Build history of the part. All positions in model axes, mm. A direction names the side the tool comes from. Round coordinates to 2 decimals unless told otherwise and drop trailing zeros. Write each loop counter-clockwise with the first axis right and the second up, starting at its lowest first coordinate (ties: lowest second). Pieces come first, ordered by that corner, then holes. Notation, with made-up numbers: (57, 75) -> (83, 75) arc R18 cw to (83, 108) -> close; hole circle Ø7 at (9.25, -37.5). An arc over 180 degrees is marked (long way). One line per question, with ' | ' between items.
from build123d import *

# Parameters (mm, degrees)
SKETCH3_W               = 36
SKETCH3_H               = 36
SKETCH3_W_2             = 20
SKETCH3_H_2             = 20
BOSS_EXTRUDE1_DEPTH     = 22
CUT_EXTRUDE1_REACH      = 57.462
SKETCH4_R               = 2.2
CUT_EXTRUDE2_DEPTH      = 56.461698495
CUT_EXTRUDE2_DEPTH_BACK = 56.461698495
SKETCH5_R               = 6.2
SKETCH6_W               = 22
SKETCH6_H               = 22
SKETCH6_R               = 6.7
BOSS_EXTRUDE2_DEPTH     = 5.4
SKETCH7_R               = 6.7
CUT_EXTRUDE3_DEPTH      = 5.4
SKETCH8_R               = 6.7
CUT_EXTRUDE4_DEPTH      = 5.4
SKETCH9_R               = 6.7
CUT_EXTRUDE5_DEPTH      = 5.4
FILLET2_R               = 2.5
FILLET3_R               = 2.5
FILLET4_R               = 2.5
SKETCH10_R              = 1.7
CUT_EXTRUDE6_DEPTH      = 56.461698535


with BuildPart() as part:
    # Sketch3 → Boss-Extrude1 (new body)
    with BuildSketch(Plane(origin=(0, 0, 0), x_dir=(1, 0, 0), z_dir=(0, 1, 0))):
        with Locations((18, -18)):
            Rectangle(SKETCH3_W, SKETCH3_H)
        with Locations((18, -18)):
            Rectangle(SKETCH3_W_2, SKETCH3_H_2, mode=Mode.SUBTRACT)
    extrude(amount=BOSS_EXTRUDE1_DEPTH)

    # Sketch4 → Cut-Extrude1 (cut, up to next)
    with BuildSketch(Plane(origin=(0, 0, 0), x_dir=(-1, 0, 0), z_dir=(0, 0, -1)), mode=Mode.PRIVATE) as cut_extrude1_sk1:
        with Locations((-16, 11)):
            Circle(SKETCH4_R)
    cut_extrude1_tool1 = extrude(cut_extrude1_sk1.sketch, amount=-CUT_EXTRUDE1_REACH, mode=Mode.PRIVATE) & part.part
    add(cut_extrude1_tool1.solids().sort_by_distance((16, 11, 0))[0], mode=Mode.SUBTRACT)

    # Sketch5 → Cut-Extrude2 (cut, two sides: drawn at the far end of the back side and taken through both)
    with BuildSketch(Plane(origin=(36, 0, 0), x_dir=(0, 0, -1), z_dir=(1, 0, 0)).offset(-CUT_EXTRUDE2_DEPTH_BACK)):
        with Locations(Location((-20, 11, 0), (0, 0, 180))):
            Circle(SKETCH5_R)
    extrude(amount=CUT_EXTRUDE2_DEPTH + CUT_EXTRUDE2_DEPTH_BACK, mode=Mode.SUBTRACT)

    # Sketch6 → Boss-Extrude2 (add)
    with BuildSketch(Plane(origin=(0, 0, 0), x_dir=(-1, 0, 0), z_dir=(0, 0, -1))):
        with Locations((-16, 11)):
            Rectangle(SKETCH6_W, SKETCH6_H)
        with Locations(Location((-16, 11, 0), (0, 0, 180))):
            Circle(SKETCH6_R, mode=Mode.SUBTRACT)
    extrude(amount=BOSS_EXTRUDE2_DEPTH)

    # Sketch7 → Cut-Extrude3 (cut)
    with BuildSketch(Plane.XY.offset(8)):
        with Locations((16, 11)):
            Circle(SKETCH7_R)
    extrude(amount=-CUT_EXTRUDE3_DEPTH, mode=Mode.SUBTRACT)

    # Sketch8 → Cut-Extrude4 (cut)
    with BuildSketch(Plane.ZY.offset(-28)):
        with Locations((20, 11)):
            Circle(SKETCH8_R)
    extrude(amount=-CUT_EXTRUDE4_DEPTH, mode=Mode.SUBTRACT)

    # Sketch9 → Cut-Extrude5 (cut)
    with BuildSketch(Plane.ZY):
        with Locations((20, 11)):
            Circle(SKETCH9_R)
    extrude(amount=-CUT_EXTRUDE5_DEPTH, mode=Mode.SUBTRACT)

    # Fillet2
    fillet2_edges = [part.edges().sort_by_distance(p)[0] for p in [
        (5, 11, -5.4),
        (27, 11, -5.4),
        (5, 11, 0),
        (27, 11, 0),
    ]]
    fillet(fillet2_edges, radius=FILLET2_R)

    # Fillet3
    fillet3_edges = [part.edges().sort_by_distance(p)[0] for p in [
        (8, 11, 28),
        (28, 11, 8),
    ]]
    fillet(fillet3_edges, radius=FILLET3_R)

    # Fillet4
    fillet4_edges = [part.edges().sort_by_distance(p)[0] for p in [
        (0, 11, 0),
        (36, 11, 0),
        (36, 11, 36),
        (0, 11, 36),
    ]]
    fillet(fillet4_edges, radius=FILLET4_R - 0.0001)  # a hair under: the kernel refuses the full size

    # Sketch10 → Cut-Extrude6 (cut, through all)
    with BuildSketch(Plane(origin=(0, 0, 0), x_dir=(-1, 0, 0), z_dir=(0, -1, 0))):
        with Locations(Location((-31.4, -4.6, 0), (0, 0, 90))):
            Circle(SKETCH10_R)
        with Locations(Location((-4.6, -4.6, 0), (0, 0, 90))):
            Circle(SKETCH10_R)
        with Locations(Location((-4.6, -31.4, 0), (0, 0, 90))):
            Circle(SKETCH10_R)
        with Locations(Location((-31.4, -31.4, 0), (0, 0, 90))):
            Circle(SKETCH10_R)
    extrude(amount=-CUT_EXTRUDE6_DEPTH, mode=Mode.SUBTRACT)


solid = part.part
(1) Slice it at C-C (x = 16). Write the cut outline in (y, z), then the cut area to 3 significant figures.
Calculated:
outline: (0, -5.4) -> (4.3, -5.4) -> (4.3, 0) -> (8.8, 0) -> (8.8, 2.6) -> (4.3, 2.6) -> (4.3, 8) -> (0, 8) -> close; (0, 28) -> (22, 28) -> (22, 36) -> (0, 36) -> close; (13.2, 0) -> (17.7, 0) -> (17.7, -5.4) -> (22, -5.4) -> (22, 8) -> (17.7, 8) -> (17.7, 2.6) -> (13.2, 2.6) -> close | area: 315 mm2
(2) Wall check: line 1 (X direction, y = 4.5, z = 31.4); line 2 (Y direction, x = 16, z = 1.3); line 3 (X direction, y = 3.75, z = 8.5). Give the ranges that are in metal, low to high. Write a range as from..to.
Calculated:
line 1: 0..2.9, 6.3..29.7, 33.1..36 | line 2: 0..8.8, 13.2..22 | line 3: 0..8, 27..36
(3) 3-axis set-ups, long thin cutter, end or side, ignore diameter. For faces 1 (the flat face through (8, 11, 13)), 2 (the cylindrical face through (4.248, 11.154, -0.713)), 3 (the flat face through (14, 9, 0)), 4 (the cylindrical face through (30.662, 17.643, 19.128)), 5 (the flat face through (31, 11, 0)): which of +Z, -Z, +X, -X, +Y, -Y reach the whole face in a straight line?
Calculated:
face 1: +Y, -Y | face 2: -Z, -X, +Y, -Y | face 3: -Z | face 4: none | face 5: -Z, +X, +Y, -Y
(4) Drop flat-ended pins along their axis: pin 1 (4.5 mm diameter, centred on x = 31, y = 12.5, fed in from -Z); pin 2 (4 mm diameter, centred on y = 14, z = 23.5, fed in from -X); pin 3 (1.5 mm diameter, centred on x = 5.5, y = 12.5, fed in from -Z). Give the stop position or say it passes through.
Calculated:
pin 1: z = -0.12 | pin 2: x = 5.4 | pin 3: z = -5.07
(5) Mould opens along Y. For faces 6 (the cylindrical face through (13.968, 10.157, 1.282)), 7 (the flat face through (18, 0, 6)), 8 (the flat face through (14, 13, 2.6)), 9 (the cylindrical face through (0.752, 11.154, 35.287)) say: pulls with the +Y half, pulls with the -Y half, needs draft (parallel to the pull), parting line crosses it, or undercut.
Calculated:
face 6: undercut | face 7: pulls with the -Y half | face 8: undercut | face 9: needs draft
(6) Slice it at B-B (z = 31.4). Write the cut outline in (x, y).
Calculated:
outline: (0, 0) -> (2.9, 0) -> (2.9, 22) -> (0, 22) -> close; (6.3, 0) -> (29.7, 0) -> (29.7, 22) -> (6.3, 22) -> close; (33.1, 0) -> (36, 0) -> (36, 22) -> (33.1, 22) -> close
(7) Slice it at A-A (x = 31.4). Write the cut outline in (y, z).
Calculated:
outline: (0, 0) -> (22, 0) -> (22, 2.9) -> (0, 2.9) -> close; (0, 6.3) -> (22, 6.3) -> (22, 29.7) -> (0, 29.7) -> close; (0, 33.1) -> (22, 33.1) -> (22, 36) -> (0, 36) -> close; hole circle Ø13.4 at (11, 20)
(8) Slice it at D-D (z = 9). Write the cut outline in (x, y).
Calculated:
outline: (0, 0) -> (8, 0) -> (8, 22) -> (0, 22) -> close; (27.5, 0) -> (36, 0) -> (36, 22) -> (27.5, 22) -> close
